```python
from build123d import *

# Parameters (mm, degrees)
SKETCH1_R           = 34.7
SKETCH1_R_2         = 1.55
SKETCH1_R_3         = 3.1
BOSS_EXTRUDE1_DEPTH = 10
FILLET2_R           = 1
FILLET3_R           = 0.8


with BuildPart() as part:
    # Sketch1 → Boss-Extrude1 (new body)
    with BuildSketch(Plane(origin=(0, 0, 0), x_dir=(1, 0, 0), z_dir=(0, 1, 0))):
        with Locations((0, -6.629356842)):
            Circle(SKETCH1_R)
        with Locations((0, 2.895643158)):
            Circle(SKETCH1_R_2, mode=Mode.SUBTRACT)
        with Locations((-8.248891971, -1.866856842)):
            Circle(SKETCH1_R_2, mode=Mode.SUBTRACT)
        with Locations((-8.248891971, -11.391856842)):
            Circle(SKETCH1_R_2, mode=Mode.SUBTRACT)
        with Locations((0, -16.154356842)):
            Circle(SKETCH1_R_2, mode=Mode.SUBTRACT)
        with Locations((8.248891971, -1.866856842)):
            Circle(SKETCH1_R_2, mode=Mode.SUBTRACT)
        with Locations((0, -6.629356842)):
            Circle(SKETCH1_R_3, mode=Mode.SUBTRACT)
        with Locations((8.248891971, -11.391856842)):
            Circle(SKETCH1_R_2, mode=Mode.SUBTRACT)
        with BuildLine():
            Line((-3.20212766, 23.299832563), (-3, 5.711226612))
            ThreePointArc((-3, 5.711226612), (-7.464872704, 3.645158986), (-10.809541326, 0.037262715))
            Line((-10.809541326, 0.037262715), (-27.755348523, 5.017558129))
            ThreePointArc((-27.755348523, 5.017558129), (-17.976421293, 17.513101141), (-3.20212766, 23.299832563))
        make_face(mode=Mode.SUBTRACT)
        with BuildLine():
            Line((2.5, 23.366642891), (3, 5.711226612))
            ThreePointArc((3, 5.711226612), (7.464872704, 3.645158986), (10.809541326, 0.037262715))
            Line((10.809541326, 0.037262715), (27.474838746, 5.664675689))
            ThreePointArc((27.474838746, 5.664675689), (17.405822307, 17.927665571), (2.5, 23.366642891))
        make_face(mode=Mode.SUBTRACT)
        Polygon((-0.875343089, 21.666642891), (0.847462288, 21.666642891), (1.251174555, 7.411226612), (-1.221162893, 7.411226612), align=None, mode=Mode.SUBTRACT)
        Polygon((12.9760283, -1.129183017), (26.640599041, 2.947088697), (27.17297518, 1.308603417), (13.740022588, -3.480515657), align=None, mode=Mode.SUBTRACT)
        with BuildLine():
            Line((29.453862476, -0.426133065), (12.663643293, -5.669076383))
            ThreePointArc((12.663643293, -5.669076383), (11.986909153, -10.825070007), (9.300423223, -15.27760105))
            Line((9.300423223, -15.27760105), (20.18251184, -28.960416285))
            ThreePointArc((20.18251184, -28.960416285), (28.62680114, -15.930768373), (29.453862476, -0.426133065))
        make_face(mode=Mode.SUBTRACT)
        Polygon((9.240789422, -17.270645929), (17.340138777, -29.006787741), (15.946359949, -30.019427334), (7.24062641, -18.723849419), align=None, mode=Mode.SUBTRACT)
        with BuildLine():
            Line((15.608663785, -32.36609352), (4.826561976, -18.376454334))
            ThreePointArc((4.826561976, -18.376454334), (0, -19.329356842), (-4.826561976, -18.376454334))
            Line((-4.826561976, -18.376454334), (-15.001360451, -32.724743113))
            ThreePointArc((-15.001360451, -32.724743113), (0.352649568, -36.727290962), (15.608663785, -32.36609352))
        make_face(mode=Mode.SUBTRACT)
        Polygon((-7.264906355, -18.706209007), (-15.923803908, -30.035815257), (-17.317582735, -29.023175665), (-9.265069366, -17.253005516), align=None, mode=Mode.SUBTRACT)
        with BuildLine():
            Line((-20.18251184, -28.960416285), (-9.680663942, -14.849742821))
            ThreePointArc((-9.680663942, -14.849742821), (-12.163791536, -10.280682009), (-12.607510846, -5.099431917))
            Line((-12.607510846, -5.099431917), (-29.453862476, -0.426133065))
            ThreePointArc((-29.453862476, -0.426133065), (-28.62680114, -15.930768373), (-20.18251184, -28.960416285))
        make_face(mode=Mode.SUBTRACT)
        Polygon((-13.730748474, -3.451972871), (-27.181590822, 1.2820872), (-26.649214682, 2.920572479), (-12.966754187, -1.10064023), align=None, mode=Mode.SUBTRACT)
    extrude(amount=BOSS_EXTRUDE1_DEPTH)

    # Fillet2
    fillet2_edges = [part.edges().sort_by_distance(p)[0] for p in [
        (15.608663785, 5, 32.36609352),
        (-29.453862476, 5, 0.426133065),
        (-20.18251184, 5, 28.960416285),
        (27.474838746, 5, -5.664675689),
        (2.5, 5, -23.366642891),
        (-3.20212766, 5, -23.299832563),
        (-27.755348523, 5, -5.017558129),
        (20.18251184, 5, 28.960416285),
        (29.453862476, 5, 0.426133065),
        (-15.001360451, 5, 32.724743113),
    ]]
    fillet(fillet2_edges, radius=FILLET2_R)

    # Fillet3
    fillet3_edges = [part.edges().sort_by_distance(p)[0] for p in [
        (15.946359949, 5, 30.019427334),
        (17.340138777, 5, 29.006787741),
        (9.240789422, 5, 17.270645929),
        (7.24062641, 5, 18.723849419),
        (-17.317582735, 5, 29.023175665),
        (-15.923803908, 5, 30.035815257),
        (-7.264906355, 5, 18.706209007),
        (-9.265069366, 5, 17.253005516),
        (-26.649214682, 5, -2.920572479),
        (-27.181590822, 5, -1.2820872),
        (-13.730748474, 5, 3.451972871),
        (-12.966754187, 5, 1.10064023),
        (-0.875343089, 5, -21.666642891),
        (-1.221162893, 5, -7.411226612),
        (1.251174555, 5, -7.411226612),
        (0.847462288, 5, -21.666642891),
        (27.17297518, 5, -1.308603417),
        (26.640599041, 5, -2.947088697),
        (12.9760283, 5, 1.129183017),
        (13.740022588, 5, 3.480515657),
    ]]
    fillet(fillet3_edges, radius=FILLET3_R)


solid = part.part
```
CAD build for the part. Positions are in the model's coordinates, mm. Round coordinates to 2 decimals unless told otherwise and drop trailing zeros. Loops run counter-clockwise (first coordinate to the right, second up) from the corner with the lowest first, then second, coordinate; pieces in that order, holes last. Notation, with made-up numbers: (16, 16.25) - (69, 16.25) arc R10 cw to (69, 21.25) - close; hole circle Ø6 at (-15.5, 17.5). An arc over 180 degrees is marked (long way). Return JSON: item names as keys, results as strings. Group by question number.
Q1. Band-saw the part on B-B on z = -11.5. Give the cut face in (x, y), plus the area to 3 significant figures.
Q2. Band-saw the part on A-A on x = -24. Give the cut face in (y, z).
Q3. Flat gauge pins, fed straight in: pin 1 Ø0.9 at (x, y) = (0, 5) entering from -Z; pin 2 Ø2 at (y, z) = (8.5, -1.5) entering from +X; pin 3 Ø2 at (y, z) = (5.5, 13.5) entering from -X; pin 4 Ø4 at (x, z) = (-24, -11.5) entering from -Y. Where does each tip first touch, or does it go through?
Q4. Drill centre lines: line 1 along Z through (x, y) = (13, 7); line 2 along Z through (x, y) = (19, 8.25); line 3 along X through (y, z) = (2.25, 8.5). Where is each one in solid material? Low to high. Write a range as [from, to].
Q5. Band-saw the part on C-C on y = 8. Give the number of separate pieces and of enclosed holes in the cut face, plus the area to 3 significant figures.
Q6. Two-plate mould, pull along X, no slides. Class faces 1 (the face through (-4.517, 4.93, -27.775)), 2 (the face through (12.01, 4.93, 10.76)): +X half, -X half, draft (parallel to the pull), parting line (faces both ways), or undercut.
Solutions:
{
 "1": {"outline": "(-29.59, 0) - (-24.03, 0) - (-24.03, 10) - (-29.59, 10) - close; (-3.07, 0) - (-1.12, 0) - (-1.12, 10) - (-3.07, 10) - close; (1.14, 0) - (2.84, 0) - (2.84, 10) - (1.14, 10) - close; (24.03, 0) - (29.59, 0) - (29.59, 10) - (24.03, 10) - close", "area": "148 mm^2"},
 "2": {"outline": "(0, -18.43) - (10, -18.43) - (10, -11.54) - (0, -11.54) - close; (0, -3.91) - (10, -3.91) - (10, -2.14) - (0, -2.14) - close; (0, -0.16) - (10, -0.16) - (10, 1.94) - (0, 1.94) - close; (0, 24.8) - (10, 24.8) - (10, 31.69) - (0, 31.69) - close"},
 "3": {"pin 1": "stops at z = -28.07", "pin 2": "stops at x = 33.96", "pin 3": "stops at x = -34.2", "pin 4": "stops at y = 0"},
 "4": {"line 1": "z = [-25.54, -20.52], [-0.78, 5.56], [19.93, 22.72], [26.2, 28.98], [33.78, 38.8]", "line 2": "z = [-22.41, -16.72], [-2.8, -0.67], [1.61, 3.69], [27.47, 35.67]", "line 3": "x = [-34.65, -30.04], [-12.56, -2.47], [2.47, 12.56], [30.04, 34.65]"},
 "5": {"separate pieces": "1", "enclosed holes": "17", "area": "1,740 mm^2"},
 "6": {"face 1": "parting line", "face 2": "undercut"}
}
